```python
from build123d import *

# Parameters (mm, degrees)
SKETCH1_R          = 59.69
SKETCH1_R_2        = 3.175
EXTRUDE1_DEPTH     = 3.175
SKETCH2_R          = 59.69
SKETCH2_R_2        = 54.9275
EXTRUDE2_DEPTH     = 3.175
CUT_EXTRUDE1_REACH = 5.175
SKETCH3_R          = 1.984375
SKETCH3_R_2        = 1.7272
SKETCH4_R          = 6.35
SKETCH4_R_2        = 3.175
EXTRUDE3_DEPTH     = 6.35


with BuildPart() as part:
    # Sketch1 → Extrude1 (new body)
    with BuildSketch(Plane(origin=(0, 0, 0), x_dir=(1, 0, 0), z_dir=(0, 1, 0))):
        Circle(SKETCH1_R)
        Circle(SKETCH1_R_2, mode=Mode.SUBTRACT)
    extrude(amount=EXTRUDE1_DEPTH)

    # Sketch2 → Extrude2 (add)
    with BuildSketch(Plane(origin=(0, 3.175, 0), x_dir=(-1, 0, 0), z_dir=(0, 1, 0))):
        Circle(SKETCH2_R)
        Circle(SKETCH2_R_2, mode=Mode.SUBTRACT)
    extrude(amount=EXTRUDE2_DEPTH)

    # Sketch3 → Cut-Extrude1 (cut, up to next)
    with BuildSketch(Plane(origin=(0, 3.175, 0), x_dir=(-1, 0, 0), z_dir=(0, 1, 0)), mode=Mode.PRIVATE) as cut_extrude1_sk1:
        with Locations((25.542528029, -23.818792725)):
            Circle(SKETCH3_R)
    cut_extrude1_tool1 = extrude(cut_extrude1_sk1.sketch, amount=-CUT_EXTRUDE1_REACH, mode=Mode.PRIVATE) & part.part
    add(cut_extrude1_tool1.solids().sort_by_distance((-25.542528, 3.175, -23.818793))[0], mode=Mode.SUBTRACT)
    # Sketch3 → Cut-Extrude1 (cut, up to next)
    with BuildSketch(Plane(origin=(0, 3.175, 0), x_dir=(-1, 0, 0), z_dir=(0, 1, 0)), mode=Mode.PRIVATE) as cut_extrude1_sk2:
        with Locations((25.542528029, 23.818792725)):
            Circle(SKETCH3_R)
    cut_extrude1_tool2 = extrude(cut_extrude1_sk2.sketch, amount=-CUT_EXTRUDE1_REACH, mode=Mode.PRIVATE) & part.part
    add(cut_extrude1_tool2.solids().sort_by_distance((-25.542528, 3.175, 23.818793))[0], mode=Mode.SUBTRACT)
    # Sketch3 → Cut-Extrude1 (cut, up to next)
    with BuildSketch(Plane(origin=(0, 3.175, 0), x_dir=(-1, 0, 0), z_dir=(0, 1, 0)), mode=Mode.PRIVATE) as cut_extrude1_sk3:
        with Locations((-34.925, 0)):
            Circle(SKETCH3_R)
    cut_extrude1_tool3 = extrude(cut_extrude1_sk3.sketch, amount=-CUT_EXTRUDE1_REACH, mode=Mode.PRIVATE) & part.part
    add(cut_extrude1_tool3.solids().sort_by_distance((34.925, 3.175, 0))[0], mode=Mode.SUBTRACT)
    # Sketch3 → Cut-Extrude1 (cut, up to next)
    with BuildSketch(Plane(origin=(0, 3.175, 0), x_dir=(-1, 0, 0), z_dir=(0, 1, 0)), mode=Mode.PRIVATE) as cut_extrude1_sk4:
        with Locations((-9.921875, 0)):
            Circle(SKETCH3_R_2)
    cut_extrude1_tool4 = extrude(cut_extrude1_sk4.sketch, amount=-CUT_EXTRUDE1_REACH, mode=Mode.PRIVATE) & part.part
    add(cut_extrude1_tool4.solids().sort_by_distance((9.921875, 3.175, 0))[0], mode=Mode.SUBTRACT)
    # Sketch3 → Cut-Extrude1 (cut, up to next)
    with BuildSketch(Plane(origin=(0, 3.175, 0), x_dir=(-1, 0, 0), z_dir=(0, 1, 0)), mode=Mode.PRIVATE) as cut_extrude1_sk5:
        with Locations((9.921875, 0)):
            Circle(SKETCH3_R_2)
    cut_extrude1_tool5 = extrude(cut_extrude1_sk5.sketch, amount=-CUT_EXTRUDE1_REACH, mode=Mode.PRIVATE) & part.part
    add(cut_extrude1_tool5.solids().sort_by_distance((-9.921875, 3.175, 0))[0], mode=Mode.SUBTRACT)

    # Sketch4 → Extrude3 (add)
    with BuildSketch(Plane(origin=(0, 3.175, 0), x_dir=(-1, 0, 0), z_dir=(0, 1, 0))):
        Circle(SKETCH4_R)
        Circle(SKETCH4_R_2, mode=Mode.SUBTRACT)
    extrude(amount=EXTRUDE3_DEPTH)


solid = part.part
```
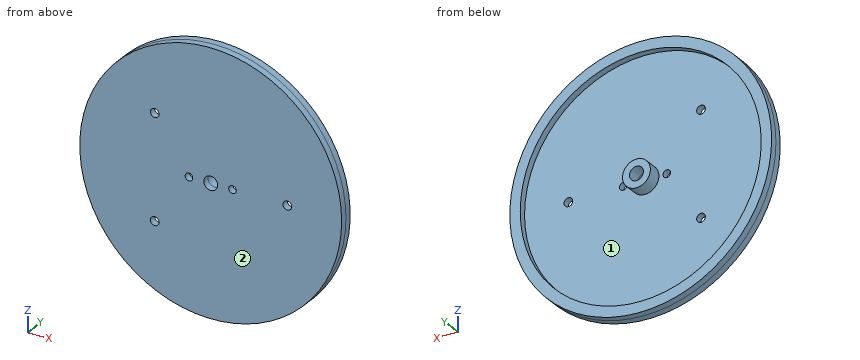
For this review, take the finished solid that the model builds, in its own axes (mm). Face numbers are marked on the shaded views. Round coordinates to 2 decimals unless told otherwise and drop trailing zeros. Write each loop counter-clockwise with the first axis right and the second up, starting at its lowest first coordinate (ties: lowest second). Pieces come first, ordered by that corner, then holes. Notation, with made-up numbers: M 65.25,-24.5 L 93.25,-24.5 A32 cw 93.25,11.5 Z; hole C -33.75,44.5 d10. An arc over 180 degrees is marked long. One line per item, written item: value. Start each with the question number.
(1) We need section A-A (z = 0). Count the separate pieces of the cut face and the enclosed holes in it, and give its area (3 significant figures).
(2) We need section D-D (z = -42). Give the boundary of the cut face in (x, y) (3 decimals).
(3) We need section C-C (y = 1.75). Give the boundary of the cut face in (x, z) (3 decimals), and give its area (3 significant figures).
(4) Wall thickness on line 1 (X direction, y = 4, z = -0.5); line 2 (Z direction, x = 0, y = 1.6) (3 decimals); line 3 (Y direction, x = 19, z = 0) (3 decimals): over which ranges is each line inside the solid? List them lowest first.
(5) Insertion check: pin 1 (1 mm diameter, centred on x = -30, y = 5, fed in from -Z); pin 2 (6 mm diameter, centred on x = 2, z = 36.5, fed in from +Y) (3 decimals); pin 3 (4 mm diameter, centred on y = 8, z = -25, fed in from -X). Each pin has a flat end and moves straight along its axis. Give the tip position at first contact, or say it passes through.
(6) The part is to be moulded in two halves that separate along X. For the marked faces 1 and 2, say which applies: released by +X, released by -X, zero draft, split by the parting line, or undercut.
Result:
1. separate pieces: 5
1. enclosed holes: 0
1. area: 395 mm²
2. outline: M -42.413,0 L 42.413,0 L 42.413,6.35 L 35.398,6.35 L 35.398,3.175 L -35.398,3.175 L -35.398,6.35 L -42.413,6.35 Z
3. outline: C 0,0 d119.38; hole C -25.543,-23.819 d3.969; hole C -25.543,23.819 d3.969; hole C -9.922,0 d3.454; hole C 0,0 d6.35; hole C 9.922,0 d3.454; hole C 34.925,0 d3.969
3. area: 11,100 mm²
4. line 1: -59.69 to -54.93, -6.33 to -3.14, 3.14 to 6.33, 54.93 to 59.69
4. line 2: -59.69 to -3.175, 3.175 to 59.69
4. line 3: 0 to 3.175
5. pin 1: z = -51.89
5. pin 2: y = 3.175
5. pin 3: x = -54.71
6. face 1: undercut
6. face 2: zero draft
